from build123d import *

# Parameters (mm, degrees)
SKETCH1_W           = 30
SKETCH1_H           = 160
BOSS_EXTRUDE1_DEPTH = 5.2
CUT_EXTRUDE1_DEPTH  = 10
FILLET1_R           = 1
BOSS_EXTRUDE2_DEPTH = 5.2
FILLET2_R           = 1


with BuildPart() as part:
    # Sketch1 → Boss-Extrude1 (new body)
    with BuildSketch(Plane(origin=(0, 0, 0), x_dir=(1, 0, 0), z_dir=(0, 1, 0))):
        with Locations((15, 80)):
            Rectangle(SKETCH1_W, SKETCH1_H)
    extrude(amount=BOSS_EXTRUDE1_DEPTH)

    # Sketch2 → Cut-Extrude1 (cut)
    with BuildSketch(Plane(origin=(0, 5.2, 0), x_dir=(1, 0, 0), z_dir=(0, 1, 0))):
        Polygon((30, 131.642135624), (22.221825407, 139.420310217), (25.686648635, 142.885133445), (30, 138.571782079), align=None)
        Polygon((30, 19.142135624), (19.393398282, 8.535533906), (0, 8.535533906), (0, 0), (30, 0), align=None)
    extrude(amount=-CUT_EXTRUDE1_DEPTH, mode=Mode.SUBTRACT)

    # Fillet1
    fillet1_edges = [part.edges().sort_by_distance(p)[0] for p in [
        (30, 2.6, -138.571782079),
        (30, 2.6, -131.642135624),
    ]]
    fillet(fillet1_edges, radius=FILLET1_R)

    # Sketch3 → Boss-Extrude2 (add)
    with BuildSketch(Plane(origin=(0, 5.2, 0), x_dir=(1, 0, 0), z_dir=(0, 1, 0))):
        Polygon((26.535176772, 15.677312396), (30, 12.212489168), (36.858935778, 19.071424946), (40.323759005, 15.606601718), (33.252691193, 8.535533906), (19.393398282, 8.535533906), align=None)
    extrude(amount=-BOSS_EXTRUDE2_DEPTH)

    # Fillet2
    fillet2_edges = [part.edges().sort_by_distance(p)[0] for p in [
        (30, 2.6, -19.142135624),
        (36.858935778, 2.6, -19.071424946),
    ]]
    fillet(fillet2_edges, radius=FILLET2_R)


solid = part.part
Source: CAD feature listing. Evaluate the final solid. Frame: model axes, mm. A direction names the side the tool comes from. Coordinates: 2 decimals unless noted, no trailing zeros. Loops run counter-clockwise (first coordinate to the right, second up) from the corner with the lowest first, then second, coordinate; pieces in that order, holes last. Notation, with made-up numbers: (31, -19) -> (60, -19) arc R31 ccw to (60, 17) -> close; hole circle Ø6 at (22.25, 35). An arc over 180 degrees is marked (long way). Answer in a Markdown table with one row per item. Add a question column.
Q1. Section B-B on y = 1.6. Return the cut outline in (x, z).
Q2. Contact query for a flat-ended pin moving along its axis: pin 1 Ø2.5 at (y, z) = (3.5, -151) entering from +X. Output: stop coordinate, or through.
Q3. Ray query, line 1 along Z through (x, y) = (25.5, 3.55); line 2 along Z through (x, y) = (26, 2.6); line 3 along X through (y, z) = (2.5, -65). Return the intervals inside material, ascending.
Q4. Section A-A on x = 24. Return the cut outline in (y, z).
Q5. Reachability of faces 1 (the face through (0, 3, -83)), 2 (the face through (30, 3, -150)), 3 (the face through (28.143, 2.636, -17.285)) from +Z, -Z, +X, -X, +Y, -Y: full face, straight path, thin tool, end or side. Return the list, or none.
Q6. Section D-D on z = -137. Return the cut outline in (x, y).
Q7. Section C-C on z = -84.5. Return the cut outline in (x, y), and give its area (3 significant figures).
Q8. Pull-direction query (Z, two-part tool) for faces 4 (the face through (28.24, 2.64, -13.97)), 5 (the face through (26.017, 2.636, -135.625)), 6 (the face through (15, 3, -160)), 7 (the face through (16, 5.2, -85)); classes: pulls with the +Z half, pulls with the -Z half, needs draft (parallel to the pull), parting line crosses it, or undercut.
Computed values:
| question | item | result |
|---|---|---|
| 1 | outline | (0, -160) -> (30, -160) -> (30, -140.99) arc R1 ccw to (28.29, -140.28) -> (25.69, -142.89) -> (22.22, -139.42) -> (29.71, -131.94) arc R1 ccw to (30, -131.23) -> (30, -19.56) arc R1 ccw to (29.71, -18.85) -> (26.54, -15.68) -> (30, -12.21) -> (36.15, -18.36) arc R1 ccw to (37.57, -18.36) -> (40.32, -15.61) -> (33.25, -8.54) -> (0, -8.54) -> close |
| 2 | pin 1 | stops at x = 30 |
| 3 | line 1 | z = -160 to -142.7, -136.14 to -8.54 |
| 3 | line 2 | z = -160 to -142.57, -135.64 to -8.54 |
| 3 | line 3 | x = 0 to 30 |
| 4 | outline | (0, -160) -> (5.2, -160) -> (5.2, -141.2) -> (0, -141.2) -> close; (0, -137.64) -> (5.2, -137.64) -> (5.2, -8.54) -> (0, -8.54) -> close |
| 5 | face 1 | +Z, -Z, -X, +Y, -Y |
| 5 | face 2 | -Z, +X, +Y, -Y |
| 5 | face 3 | +Y, -Y |
| 6 | outline | (0, 0) -> (24.64, 0) -> (24.64, 5.2) -> (0, 5.2) -> close |
| 7 | outline | (0, 0) -> (30, 0) -> (30, 5.2) -> (0, 5.2) -> close |
| 7 | area | 156 mm^2 |
| 8 | face 4 | undercut |
| 8 | face 5 | undercut |
| 8 | face 6 | pulls with the -Z half |
| 8 | face 7 | needs draft |
